Input: part model. Units: mm. Frame: model coordinates. Face numbers are marked on the shaded views. A direction names the side the tool comes from. Round coordinates to 2 decimals unless told otherwise and drop trailing zeros. Order: outer loops, then holes, each group sorted by start corner. A loop starts at its lowest first (then second) coordinate and runs counter-clockwise, first axis right, second up.
Item 1: Line query: L1, parallel to Y at x = -0.5, z = 0; L2, parallel to Y at x = -4, z = -0.5; L3, parallel to Z at x = 2, y = 0.75. Output: solid intervals per line, ascending.
Item 2: Cut plane A-A on y = 2.5. Output: boundary loops of the cut face in (x, z).
Item 3: Cut plane B-B on z = 7.5. Output: boundary loops of the cut face in (x, y), then the cut area to 3 significant figures.
Item 4: Cut plane D-D on y = -2.5. Output: boundary loops of the cut face in (x, z), then the cut area to 3 significant figures.
Item 5: Reachability of the marked faces 4, 5 and 6 from +Z, -Z, +X, -X, +Y, -Y: full face, straight path, thin tool, end or side. Return the list, or none.
Item 6: First-contact query: pin 1 (3 mm diameter, centred on x = 1.5, z = 14, fed in from +Y); pin 2 (4 mm diameter, centred on x = -2, z = 11, fed in from -Y); pin 3 (1.3 mm diameter, centred on x = -4.5, z = -1, fed in from +Y). Flat tips, straight axial feed; report the tip coordinate or a pass-through.
Item 7: Cut plane C-C on x = -0.5. Output: boundary loops of the cut face in (y, z), then the cut area to 3 significant figures.
Item 8: Mould query, pull axis X, two halves, no side actions, for the marked faces 1, 2 and 3. Classes: released by +X, released by -X, zero draft, split by the parting line, or undercut.
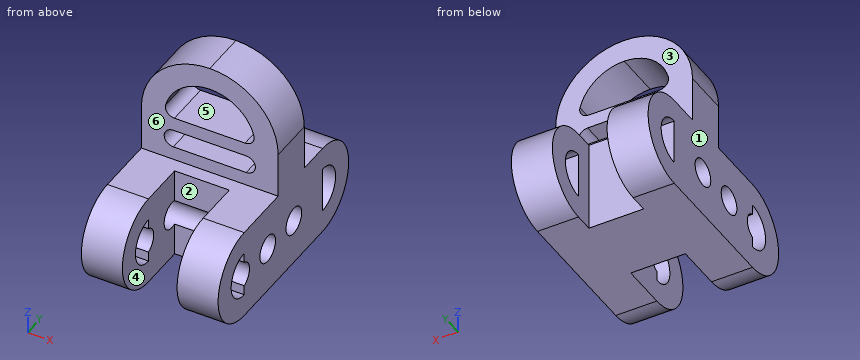
```python
from build123d import *

# Parameters (mm, degrees)
SKETCH2_R           = 5
SKETCH2_R_2         = 2.5
BOSS_EXTRUDE2_DEPTH = 7.5
SKETCH3_W           = 6
SKETCH3_H           = 10
CUT_EXTRUDE1_DEPTH  = 7.5
MIRROR1_START       = -3
MIRROR1_OUTLINE_W   = 5
MIRROR1_OUTLINE_H   = 10
MIRROR1_DEPTH       = 6
MIRROR1_START_2     = -7.5
MIRROR1_2_OUTLINE_W = 5
MIRROR1_2_OUTLINE_H = 10
MIRROR1_2_DEPTH     = 15
MIRROR1_3_DEPTH     = 4.5
MIRROR1_START_3     = 3
MIRROR1_4_DEPTH     = 4.5
SKETCH4_R           = 1.5
CUT_EXTRUDE2_DEPTH  = 15
SKETCH6_W           = 6
SKETCH6_H           = 2
CUT_EXTRUDE3_DEPTH  = 15
SKETCH7_W           = 15
SKETCH7_H           = 5
BOSS_EXTRUDE3_DEPTH = 5
BOSS_EXTRUDE4_DEPTH = 5
FILLET1_R           = 1
CUT_EXTRUDE4_DEPTH  = 5


# Read off the part's stored shape, not the designer's step: Mirror1
with BuildPart() as part:
    # Sketch2 → Boss-Extrude2 (new, symmetric)
    # profile 1 of 2: a face of its own
    with BuildSketch(Plane(origin=(0, 0, 0), x_dir=(0, 0, -1), z_dir=(1, 0, 0))):
        with Locations((0, 8)):
            Circle(SKETCH2_R)
        with Locations((0, 8)):
            Circle(SKETCH2_R_2, mode=Mode.SUBTRACT)
    # profile 2 of 2: a face of its own
    with BuildSketch(Plane(origin=(0, 0, 0), x_dir=(0, 0, -1), z_dir=(1, 0, 0))):
        with BuildLine():
            Line((-5, 8), (-5, -7))
            Line((-5, -7), (5, -7))
            Line((5, -7), (5, 8))
            ThreePointArc((5, 8), (0, 3), (-5, 8))
        make_face()
    extrude(amount=BOSS_EXTRUDE2_DEPTH, both=True)

    # Sketch3 → Cut-Extrude1 (cut, symmetric)
    with BuildSketch(Plane.XY):
        with Locations((0, 8)):
            Rectangle(SKETCH3_W, SKETCH3_H)
    extrude(amount=CUT_EXTRUDE1_DEPTH, both=True, mode=Mode.SUBTRACT)

    # Mirror1 outline → Mirror1 (cut)
    with BuildSketch(Plane.YZ.offset(MIRROR1_START)):
        with Locations((-4.5, 0)):
            Rectangle(MIRROR1_OUTLINE_W, MIRROR1_OUTLINE_H)
    extrude(amount=MIRROR1_DEPTH, mode=Mode.SUBTRACT)

    # Mirror1 2 outline → Mirror1 2 (add)
    with BuildSketch(Plane.YZ.offset(MIRROR1_START_2)):
        with Locations((5.5, 0)):
            Rectangle(MIRROR1_2_OUTLINE_W, MIRROR1_2_OUTLINE_H)
    extrude(amount=MIRROR1_2_DEPTH)

    # Mirror1 3 outline → Mirror1 3 (add)
    with BuildSketch(Plane.YZ.offset(MIRROR1_START_2)):
        with BuildLine():
            Line((-7, 2.5), (-7, 5))
            ThreePointArc((-7, 5), (-12, 0), (-7, -5))
            Line((-7, -5), (-7, -2.5))
            ThreePointArc((-7, -2.5), (-9.5, 0), (-7, 2.5))
        make_face()
    extrude(amount=MIRROR1_3_DEPTH)

    # Mirror1 4 outline → Mirror1 4 (add)
    with BuildSketch(Plane.YZ.offset(MIRROR1_START_3)):
        with BuildLine():
            Line((-7, 2.5), (-7, 5))
            ThreePointArc((-7, 5), (-12, 0), (-7, -5))
            Line((-7, -5), (-7, -2.5))
            ThreePointArc((-7, -2.5), (-9.5, 0), (-7, 2.5))
        make_face()
    extrude(amount=MIRROR1_4_DEPTH)

    # Sketch4 → Cut-Extrude2 (cut)
    with BuildSketch(Plane(origin=(7.5, 0, 0), x_dir=(0, 0, -1), z_dir=(1, 0, 0))):
        with Locations((0, 2.5)):
            Circle(SKETCH4_R)
        with Locations((0, -2.5)):
            Circle(SKETCH4_R)
        with Locations((0, -7.5)):
            Circle(SKETCH4_R)
    extrude(amount=-CUT_EXTRUDE2_DEPTH, mode=Mode.SUBTRACT)

    # Sketch6 → Cut-Extrude3 (cut)
    with BuildSketch(Plane.XY.offset(5)):
        with Locations((0, 7)):
            Rectangle(SKETCH6_W, SKETCH6_H)
    extrude(amount=-CUT_EXTRUDE3_DEPTH, mode=Mode.SUBTRACT)

    # Sketch7 → Boss-Extrude3 (add)
    with BuildSketch(Plane.XY.offset(5)):
        with Locations((0, 2)):
            Rectangle(SKETCH7_W, SKETCH7_H)
    extrude(amount=BOSS_EXTRUDE3_DEPTH)

    # Sketch8 → Boss-Extrude4 (add)
    with BuildSketch(Plane(origin=(0, 4.5, 0), x_dir=(1, 0, 0), z_dir=(0, 1, 0))):
        with BuildLine():
            ThreePointArc((5, -10), (3.535533906, -13.535533906), (0, -15))
            Line((0, -15), (0, -17.5))
            ThreePointArc((0, -17.5), (5.303300859, -15.303300859), (7.5, -10))
            Line((7.5, -10), (5, -10))
        make_face()
        with BuildLine():
            Line((0, -17.5), (0, -15))
            ThreePointArc((0, -15), (-3.535533906, -13.535533906), (-5, -10))
            Line((-5, -10), (-7.5, -10))
            ThreePointArc((-7.5, -10), (-5.303300859, -15.303300859), (0, -17.5))
        make_face()
    extrude(amount=-BOSS_EXTRUDE4_DEPTH)

    # Fillet1
    fillet1_edges = [part.edges().sort_by_distance(p)[0] for p in [
        (-5, 2, 10),
        (5, 2, 10),
    ]]
    fillet(fillet1_edges, radius=FILLET1_R)

    # Sketch9 → Cut-Extrude4 (cut)
    with BuildSketch(Plane(origin=(0, 4.5, 0), x_dir=(1, 0, 0), z_dir=(0, 1, 0))):
        with BuildLine():
            Line((-4, -6.5), (4, -6.5))
            ThreePointArc((4, -6.5), (5, -7.5), (4, -8.5))
            Line((4, -8.5), (-4, -8.5))
            ThreePointArc((-4, -8.5), (-5, -7.5), (-4, -6.5))
        make_face()
    extrude(amount=-CUT_EXTRUDE4_DEPTH, mode=Mode.SUBTRACT)


solid = part.part
```
From the geometry:
1. L1: y = -1 to 1, 4 to 6
1. L2: y = -11.97 to -9.45, -6.09 to -3.91, -1.09 to 1.09, 3.91 to 8, 10.45 to 12.97
1. L3: z = -5 to 6.5, 8.5 to 10, 14.58 to 17.23
2. outline: (-7.5, -5) - (7.5, -5) - (7.5, -1.5) - (-7.5, -1.5) - close; (-7.5, 1.5) - (7.5, 1.5) - (7.5, 10) arc R7.5 ccw to (-7.5, 10) - close; hole (-4.84, 11.25) arc R1 ccw to (-3.87, 10) - (3.87, 10) arc R1 ccw to (4.84, 11.25) arc R5 ccw to start; hole (-4, 6.5) - (4, 6.5) arc R1 ccw to (4, 8.5) - (-4, 8.5) arc R1 ccw to start
3. outline: (-7.5, -0.5) - (-5, -0.5) - (-5, 4.5) - (-7.5, 4.5) - close; (5, -0.5) - (7.5, -0.5) - (7.5, 4.5) - (5, 4.5) - close
3. area: 25.0 mm2
4. outline: (-7.5, -5) - (-3, -5) - (-3, -1.5) - (-7.5, -1.5) - close; (-7.5, 1.5) - (-3, 1.5) - (-3, 5) - (-7.5, 5) - close; (3, -5) - (7.5, -5) - (7.5, -1.5) - (3, -1.5) - close; (3, 1.5) - (7.5, 1.5) - (7.5, 5) - (3, 5) - close
4. area: 63.0 mm2
5. face 4: +Z, -Z, -Y
5. face 5: +Y, -Y
5. face 6: +Z, +X, -X, -Y
6. pin 1: stops at y = 4.5
6. pin 2: stops at y = -0.5
6. pin 3: stops at y = 12.99
7. outline: (-2, -5) - (6, -5) - (6, 5) - (4.5, 5) - (4.5, 6.5) - (-0.5, 6.5) - (-0.5, 5) - (-2, 5) - (-2, 1.41) arc R1.5 cw to (-2, -1.41) - close; (-0.5, 8.5) - (4.5, 8.5) - (4.5, 10) - (-0.5, 10) - close; (-0.5, 14.97) - (4.5, 14.97) - (4.5, 17.48) - (-0.5, 17.48) - close; hole circle Ø3 at (2.5, 0)
7. area: 98.4 mm2
8. face 1: released by -X
8. face 2: undercut
8. face 3: zero draft
